Can you work these out from the drawing? Everything is in mm from the part's minimum corner. Coordinates: 2 decimals unless noted, no trailing zeros. Order: outer loops, then holes, each group sorted by start corner. A loop starts at its lowest first (then second) coordinate and runs counter-clockwise, first axis right, second up. Notation, with made-up numbers: (57.25, 37) -> (99.25, 37) arc R17 cw to (99.25, 64) -> close; hole circle Ø9 at (2, 9). An arc over 180 degrees is marked (long way). Return JSON: item names as keys, results as strings. Group by question number.
1) For pin 1 (1.5 mm diameter, centred on x = 29.5, y = 4, fed in from -Z); pin 2 (3 mm diameter, centred on y = 3.5, z = 1.5, fed in from +X); pin 3 (3 mm diameter, centred on y = 4.5, z = 2.5, fed in from -X); pin 4 (3 mm diameter, centred on x = 8, y = 1.5, fed in from +Z), each with a flat end and sliding along its axis, tell me the tip position at first contact or that it passes through.
2) If we section it at A-A, the plane y = 2: Please give me the cut outline in (x, z), then the cut area to 3 significant figures.
3) If I drill on probe 1 along Z at (x, y) = (113, 2.5); probe 2 along X at (y, z) = (3.25, 8.5), over which ranges is the centre line in solid material (lowest first)? Write a range as from..to.
4) If we section it at C-C, the plane z = 23.75: Please give me the cut outline in (x, y).
5) If we section it at B-B, the plane x = 10: Please give me the cut outline in (y, z).
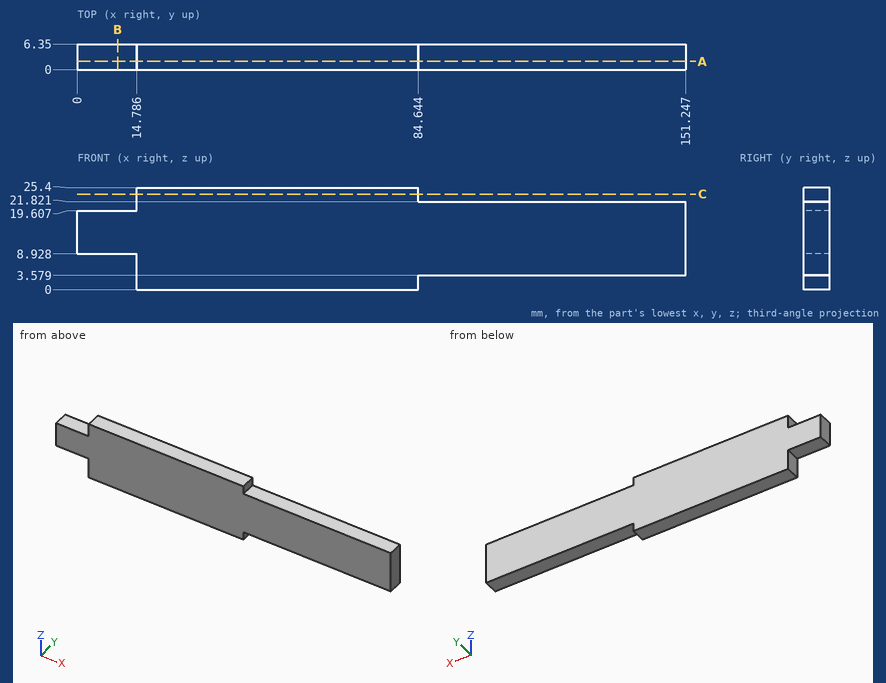
Result sheet:
{
 "1": {"pin 1": "stops at z = 0", "pin 2": "stops at x = 84.64", "pin 3": "stops at x = 14.79", "pin 4": "stops at z = 19.61"},
 "2": {"outline": "(0, 8.93) -> (14.79, 8.93) -> (14.79, 0) -> (84.64, 0) -> (84.64, 3.58) -> (151.25, 3.58) -> (151.25, 21.82) -> (84.64, 21.82) -> (84.64, 25.4) -> (14.79, 25.4) -> (14.79, 19.61) -> (0, 19.61) -> close", "area": "3,150 mm2"},
 "3": {"probe 1": "z = 3.58..21.82", "probe 2": "x = 14.79..151.25"},
 "4": {"outline": "(14.79, 0) -> (84.64, 0) -> (84.64, 6.35) -> (14.79, 6.35) -> close"},
 "5": {"outline": "(0, 8.93) -> (6.35, 8.93) -> (6.35, 19.61) -> (0, 19.61) -> close"}
}
